Autodesk Inventor part; units mm, degrees
ref_plane "YZ Plane" through (0, 0, 0) normal (1, 0, 0) x (0, 1, 0)
ref_plane "XZ Plane" through (0, 0, 0) normal (0, 1, 0) x (-1, 0, 0)
ref_plane "XY Plane" through (0, 0, 0) normal (0, 0, 1) x (1, 0, 0)
sketch "Sketch1" plane through (0, 0, 0) normal (0, 1, 0) x (-1, 0, 0)
  line L0 (0, 0) -> (10, 0)
  line L1 (10, 0) -> (10, -9)
  line L2 (10, -9) -> (0, -9)
  line L3 (0, -9) -> (0, 0)
  line L4 (10, 0) -> (16.35, 0)
  line L5 (16.35, 0) -> (16.35, -22.225)
  line L6 (16.35, -22.225) -> (10, -22.225)
  line L7 (10, -22.225) -> (10, 0)
  line L8 (0, 0) -> (-12.7, 0)
  line L9 (-12.7, 0) -> (-12.7, -22.225)
  line L10 (-12.7, -22.225) -> (0, -22.225)
  line L11 (0, -22.225) -> (0, 0)
  point P0 (0, -9)
  point P1 (10, -9)
  dimension "d0" = 10
  dimension "d1" = 9
  dimension "d2" = 6.35
  dimension "d3" = 22.225
  dimension "d4" = 22.225
  dimension "d5" = 12.7
revolve "Revolution1" add sketch "Sketch1" angle 360 about axis through (0, 0, 0) along (-1, 0, 0)
equation "\"d4\" = d3"
properties part number "Temp Sprocket" material "Nylon 6/6"
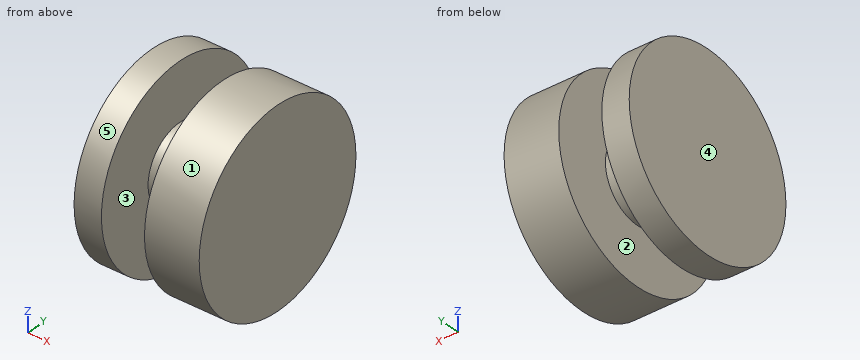
The listing builds one solid part. Answer for the finished solid, in the listing's coordinates (mm). Face numbers are marked on the shaded views. A direction names the side the tool comes from. Give positions to 0.01 mm unless a question says otherwise; leave off trailing zeros. Order: outer loops, then holes, each group sorted by start corner. A loop starts at its lowest first (then second) coordinate and runs counter-clockwise, first axis right, second up. Notation, with made-up numbers: M 60,87 L 81,87 A20 ccw 81,109 Z; hole C 32,15 d11. An arc over 180 degrees is marked long. Put each result on its own line as item: value. Start each with the question number.
Item 1: The part is cut by section A-A, the plane y = 0. Determine the outline of the cut face in (x, z) (3 decimals), and give its area (3 significant figures).
Item 2: Which of the six approach directions +Z, -Z, +X, -X, +Y, -Y give full straight-line access (tool end or side, diameter ignored) to the marked faces 1 and 2?
Item 3: Flat-ended cylindrical pins translate along their axes: P1, Ø6, axis at x = 8.5, y = -8.5, coming from the -Z side; P2, Ø8, axis at x = -1, y = 6.5, coming from the +Z side; P3, Ø5, axis at x = 0, y = 0.5, coming from the -Z side (3 decimals). Find the tip coordinate at first contact, or state that the pin passes through.
Item 4: For a pull along X with two mould halves and no side action, classify the marked faces 3, 4 and 5 as +X half, -X half, draft (parallel to the pull), parting line (faces both ways), or undercut.
Item 5: The part is cut by section C-C, the plane y = 17. Determine the outline of the cut face in (x, z).
Item 6: Find the intervals of material crossed by line 1 along X through (y, z) = (11, -16.5); line 2 along Z through (x, y) = (-8, 2.5); line 3 along Z through (x, y) = (5.5, 7), in increasing order.
Item 7: The part is cut by section D-D, the plane z = -11. Determine the outline of the cut face in (x, y).
Answer key:
1. outline: M -16.35,-22.225 L -10,-22.225 L -10,-9 L 0,-9 L 0,-22.225 L 12.7,-22.225 L 12.7,22.225 L 0,22.225 L 0,9 L -10,9 L -10,22.225 L -16.35,22.225 Z
1. area: 1,030 mm²
2. face 1: +X, -X
2. face 2: none
3. P1: stops at z = -21.53
3. P2: stops at z = 22.07
3. P3: stops at z = -22.225
4. face 3: undercut
4. face 4: -X half
4. face 5: draft
5. outline: M -16.35,-14.32 L -10,-14.32 L -10,14.32 L -16.35,14.32 Z; M 0,-14.32 L 12.7,-14.32 L 12.7,14.32 L 0,14.32 Z
6. line 1: x = -16.35 to -10, 0 to 12.7
6. line 2: z = -8.65 to 8.65
6. line 3: z = -21.09 to 21.09
7. outline: M -16.35,-19.31 L -10,-19.31 L -10,19.31 L -16.35,19.31 Z; M 0,-19.31 L 12.7,-19.31 L 12.7,19.31 L 0,19.31 Z
